```python
from build123d import *

# Parameters (mm, degrees)
BOSS_EXTRUDE1_DEPTH = 6
SKETCH6_R           = 3
CUT_EXTRUDE2_DEPTH  = 144
SKETCH7_R           = 3
CUT_EXTRUDE3_DEPTH  = 144


with BuildPart() as part:
    # Sketch5 → Boss-Extrude1 (new body)
    with BuildSketch(Plane.XY):
        with BuildLine():
            Line((0, 123.2), (0, 130))
            ThreePointArc((0, 130), (-91.923881554, 91.923881554), (-130, 0))
            Line((-130, 0), (-123.2, 0))
            ThreePointArc((-123.2, 0), (-87.115555442, 87.115555442), (0, 123.2))
        make_face()
    extrude(amount=BOSS_EXTRUDE1_DEPTH)

    # Sketch6 → Cut-Extrude2 (cut)
    with BuildSketch(Plane(origin=(0, 0, 0), x_dir=(1, 0, 0), z_dir=(0, 1, 0))):
        with Locations((0, -3)):
            Circle(SKETCH6_R)
    extrude(amount=CUT_EXTRUDE2_DEPTH, mode=Mode.SUBTRACT)

    # Sketch7 → Cut-Extrude3 (cut)
    with BuildSketch(Plane(origin=(0, 0, 0), x_dir=(0, 0, -1), z_dir=(1, 0, 0))):
        with Locations((-3, 0)):
            Circle(SKETCH7_R)
    extrude(amount=-CUT_EXTRUDE3_DEPTH, mode=Mode.SUBTRACT)


solid = part.part
```
Work out the finished part from the listing and answer in its coordinate system (mm). Round coordinates to 2 decimals unless told otherwise and drop trailing zeros. Order: outer loops, then holes, each group sorted by start corner. A loop starts at its lowest first (then second) coordinate and runs counter-clockwise, first axis right, second up.
Q1. The mould has two halves that part along Z. Classify faces 1 (the cylindrical face through (-127, 3, 3)), 2 (the flat face through (-89, 89, 6)), 3 (the flat face through (-89, 89, 0)): pulls with the +Z half, pulls with the -Z half, needs draft (parallel to the pull), parting line crosses it, or undercut.
Solution:
face 1: undercut
face 2: pulls with the +Z half
face 3: pulls with the -Z half
Q2. Find the intervals of material crossed by line 1 along Y through (x, z) = (-43, 4.5); line 2 along Y through (x, z) = (-95, 4.75); line 3 along X through (y, z) = (37, 2), in increasing order.
Solution:
line 1: y = 115.45 to 122.68
line 2: y = 78.44 to 88.74
line 3: x = -124.62 to -117.51
Q3. A cutting plane is placed at A-A, the plane x = -42.5. Determine the outline of the cut face in (y, z), then the cut area to 3 significant figures.
Solution:
outline: (115.64, 0) - (122.86, 0) - (122.86, 6) - (115.64, 6) - close
area: 43.3 mm2
Q4. A cutting plane is placed at B-B, the plane z = 5. Determine the outline of the cut face in (x, y), then the cut area to 3 significant figures.
Solution:
outline: (-129.98, 2.24) - (-123.18, 2.24) arc R123.2 cw to (-2.24, 123.18) - (-2.24, 129.98) arc R130 ccw to start
area: 1,320 mm2
